The figure shows three views and two pictorial views of one solid part (mm, origin at its lowest corner). Answer the questions. A direction names the side the tool comes from. Round coordinates to 2 decimals unless told otherwise and drop trailing zeros. Order: outer loops, then holes, each group sorted by start corner. A loop starts at its lowest first (then second) coordinate and runs counter-clockwise, first axis right, second up. Notation, with made-up numbers: (22, 57) -> (65, 57) arc R29 cw to (65, 91) -> close; hole circle Ø8 at (-16.5, 47.25). An arc over 180 degrees is marked (long way). Answer as a JSON object with one key per item and string values. Group by question number.
Item 1: Given P1, Ø4, axis at x = 7, y = 3.5, coming from the +Z side; P2, Ø1, axis at y = 6, z = 2, coming from the +X side; P3, Ø2, axis at y = 1, z = 12, coming from the +X side; P4, Ø2, axis at y = 6, z = 3.5, coming from the +X side, each flat-ended and moving along its own axis, determine where each tip first touches the part or whether it passes through.
Item 2: Section B-B, the plane x = 7 is taken. Write down the section's boundary in (y, z) (3 decimals), plus the area to 3 significant figures.
Item 3: Section C-C, the plane y = 3.5 is taken. Write down the section's boundary in (x, z), plus the area to 3 significant figures.
Item 4: For the marked faces 1 and 2, determine the directions among +Z, -Z, +X, -X, +Y, -Y from which every point of the face is accessible in a straight line to the end or side of a thin tool.
Item 5: Section A-A, the plane z = 7 is taken. Write down the section's boundary in (x, y) (3 decimals), plus the area to 3 significant figures.
Item 6: Consider probe 1 along Y at (x, z) = (1.2, 7); probe 2 along X at (y, z) = (4, 13.25); probe 3 along Z at (x, y) = (6.75, 0.75). Determine where each line is inside the solid, lowest interval first. Write a range as from..to.
Item 7: Section D-D, the plane y = 1 is taken. Write down the section's boundary in (x, z).
Item 8: The mould has two halves that part along Z. Classify the marked faces 3, 4 and 5: pulls with the +Z half, pulls with the -Z half, needs draft (parallel to the pull), parting line crosses it, or undercut.
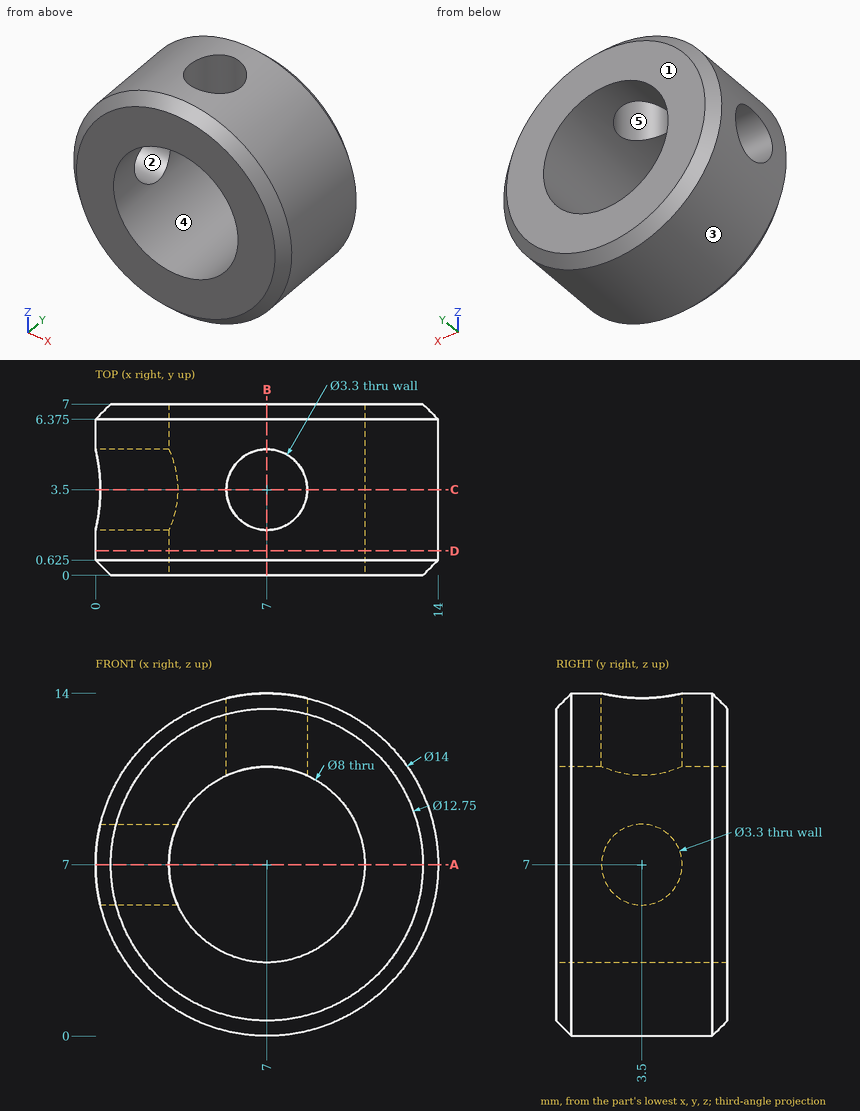
Values found:
{
 "1": {"P1": "z = 14", "P2": "x = 12.36", "P3": "x = 12.74", "P4": "x = 13.54"},
 "2": {"outline": "(0, 0.625) -> (0.625, 0) -> (6.375, 0) -> (7, 0.625) -> (7, 3) -> (0, 3) -> close; (0, 11) -> (1.85, 11) -> (1.85, 14) -> (0.625, 14) -> (0, 13.375) -> close; (5.15, 11) -> (7, 11) -> (7, 13.375) -> (6.375, 14) -> (5.15, 14) -> close", "area": "31.3 mm2"},
 "3": {"outline": "(0.2, 5.35) arc R7 ccw (long way) to (8.65, 13.8) -> (8.65, 10.64) arc R4 cw (long way) to (3.36, 5.35) -> close; (0.2, 8.65) -> (3.36, 8.65) arc R4 cw to (5.35, 10.64) -> (5.35, 13.8) arc R7 ccw to start", "area": "83.5 mm2"},
 "4": {"face 1": "+Z, -Z, +X, -X, +Y", "face 2": "-X"},
 "5": {"outline": "(0, 0.625) -> (0.625, 0) -> (3, 0) -> (3, 1.85) -> (0, 1.85) -> close; (0, 5.15) -> (3, 5.15) -> (3, 7) -> (0.625, 7) -> (0, 6.375) -> close; (11, 0) -> (13.375, 0) -> (14, 0.625) -> (14, 6.375) -> (13.375, 7) -> (11, 7) -> close", "area": "31.3 mm2"},
 "6": {"probe 1": "0..1.85, 5.15..7", "probe 2": "3.85..5.43, 8.57..10.15", "probe 3": "0..3.01, 10.99..14"},
 "7": {"outline": "circle Ø14 at (7, 7); hole circle Ø8 at (7, 7)"},
 "8": {"face 3": "parting line crosses it", "face 4": "undercut", "face 5": "needs draft"}
}
